Part print with two shaded views. Sizes in mm from the minimum x, y, z corner. A direction names the side the tool comes from. Round coordinates to 2 decimals unless told otherwise and drop trailing zeros. Order: outer loops, then holes, each group sorted by start corner. A loop starts at its lowest first (then second) coordinate and runs counter-clockwise, first axis right, second up. Notation, with made-up numbers: M -16,13.25 L 23,13.25 A27 cw 23,51.25 Z; hole C -23.75,76.25 d10. An arc over 180 degrees is marked long. Put each result on its own line as item: value.
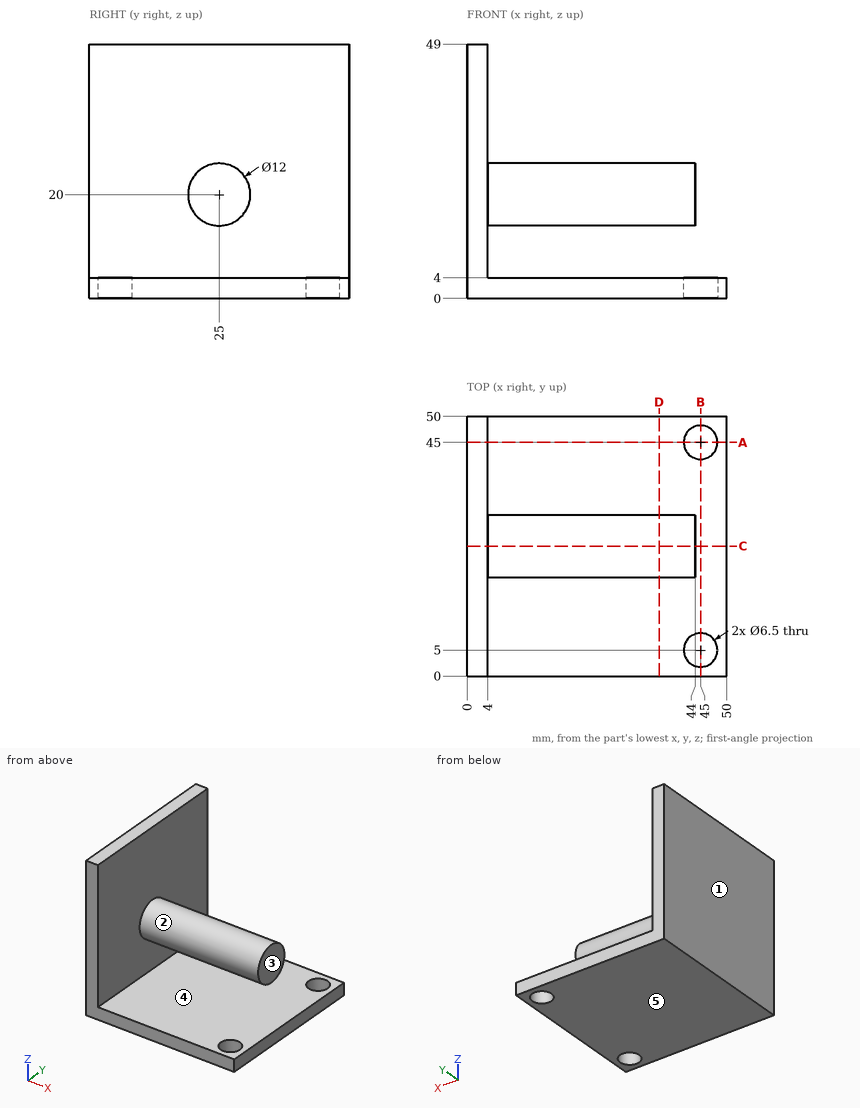
Item 1: Tool access for the marked faces 1 and 2: list every direction of +Z, -Z, +X, -X, +Y, -Y with a clear straight run to the whole face (end or side of a thin tool).
Answers below:
face 1: +Z, -Z, -X, +Y, -Y
face 2: +X
Item 2: Band-saw the part on B-B on x = 45. Give the cut face in (y, z).
Answers below:
outline: M 0,0 L 1.75,0 L 1.75,4 L 0,4 Z; M 8.25,0 L 41.75,0 L 41.75,4 L 8.25,4 Z; M 48.25,0 L 50,0 L 50,4 L 48.25,4 Z
Item 3: Probe line 1 along Y through (x, z) = (45, 0.8); line 2 along X through (y, z) = (42, 32); line 3 along Z through (x, y) = (13, 22.5). List the from-to ranges inside material, lowest first. Write a range as [from, to].
Answers below:
line 1: [0, 1.75], [8.25, 41.75], [48.25, 50]
line 2: [0, 4]
line 3: [0, 4], [14.55, 25.45]
Item 4: Band-saw the part on C-C on y = 25. Give the cut face in (x, z), and give its area (3 significant figures).
Answers below:
outline: M 0,0 L 50,0 L 50,4 L 4,4 L 4,14 L 44,14 L 44,26 L 4,26 L 4,49 L 0,49 Z
area: 860 mm²
Item 5: Pin check, flat tips, straight feed: P1, Ø8, axis at x = 33.5, z = 18, coming from the -Y side; P2, Ø2, axis at x = 40.5, y = 44.5, coming from the +Z side; P3, Ø13, axis at y = 27.5, z = 21.5, coming from the +X side; P4, Ø6, axis at x = 45, y = 45, coming from the -Z side. Stop position of each tip, or through.
Answers below:
P1: y = 19
P2: z = 4
P3: x = 44
P4: through
Item 6: Band-saw the part on D-D on x = 37. Give the cut face in (y, z).
Answers below:
outline: M 0,0 L 50,0 L 50,4 L 0,4 Z; C 25,20 d12
Item 7: Mould opens along Z. For the marked faces 3, 4 and 5 say: pulls with the +Z half, pulls with the -Z half, needs draft (parallel to the pull), parting line crosses it, or undercut.
Answers below:
face 3: needs draft
face 4: undercut
face 5: pulls with the -Z half
Item 8: Band-saw the part on A-A on y = 45. Give the cut face in (x, z).
Answers below:
outline: M 0,0 L 41.75,0 L 41.75,4 L 4,4 L 4,49 L 0,49 Z; M 48.25,0 L 50,0 L 50,4 L 48.25,4 Z
